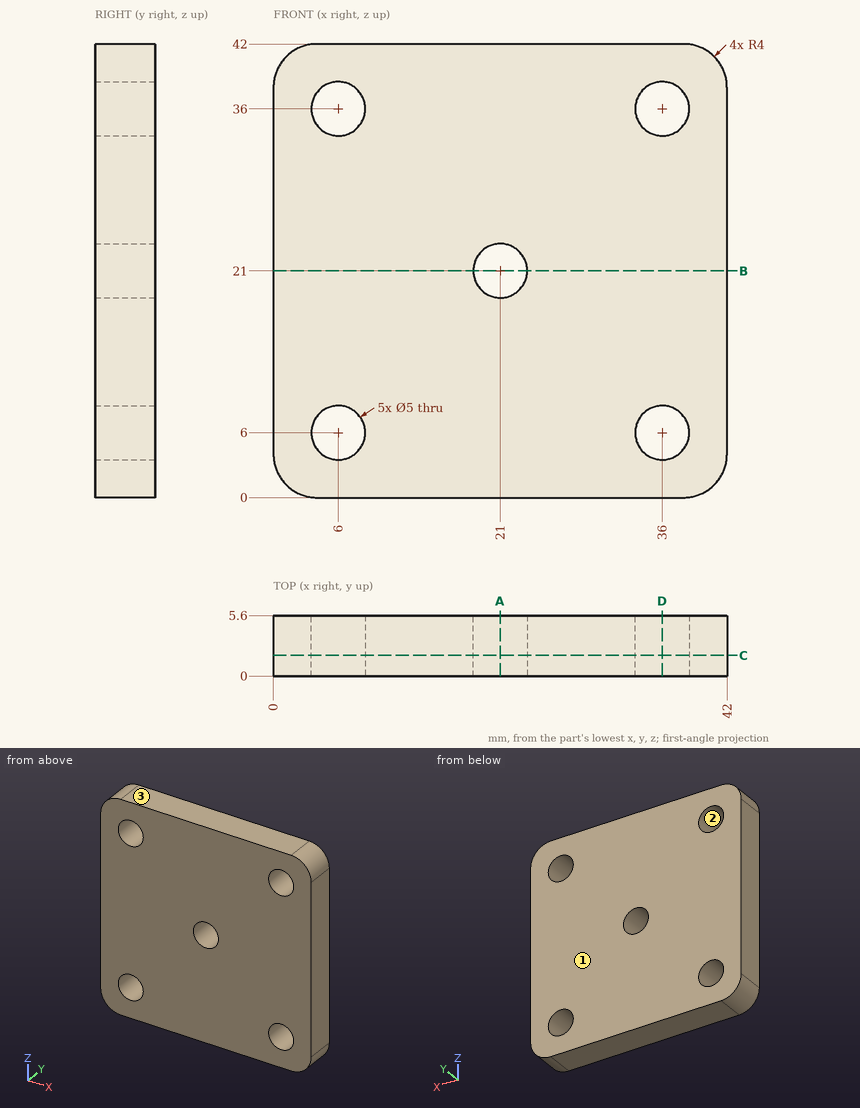
The figure shows three views and two pictorial views of one solid part (mm, origin at its lowest corner). Answer the questions. Round coordinates to 2 decimals unless told otherwise and drop trailing zeros. Write each loop counter-clockwise with the first axis right and the second up, starting at its lowest first coordinate (ties: lowest second). Pieces come first, ordered by that corner, then holes. Notation, with made-up numbers: M 54.5,-25.5 L 66.5,-25.5 A15 cw 66.5,-10.5 Z; hole C 75.25,-40 d10. An arc over 180 degrees is marked long. Use a Markdown table: item, result.
1) The part is cut by section D-D on x = 36. Give the vertices of the cut face in (y, z).
Taken from the geometry:
| item | result |
|---|---|
| outline | M 0,0 L 5.6,0 L 5.6,3.5 L 0,3.5 Z; M 0,8.5 L 5.6,8.5 L 5.6,33.5 L 0,33.5 Z; M 0,38.5 L 5.6,38.5 L 5.6,42 L 0,42 Z |
2) Determine the mould class of the marked faces 1, 2 and 3 for opening direction Z: pulls with the +Z half, pulls with the -Z half, needs draft (parallel to the pull), parting line crosses it, or undercut.
Taken from the geometry:
| item | result |
|---|---|
| face 1 | needs draft |
| face 2 | undercut |
| face 3 | pulls with the +Z half |
3) The part is cut by section C-C on y = 1.9. Give the vertices of the cut face in (x, z), plus the area to 3 significant figures.
Taken from the geometry:
| item | result |
|---|---|
| outline | M 0,4 A4 ccw 4,0 L 38,0 A4 ccw 42,4 L 42,38 A4 ccw 38,42 L 4,42 A4 ccw 0,38 Z; hole C 6,6 d5; hole C 6,36 d5; hole C 21,21 d5; hole C 36,6 d5; hole C 36,36 d5 |
| area | 1,650 mm2 |
4) Consider line 1 (Z direction, x = 36, y = 4.65); line 2 (X direction, y = 0.85, z = 8); line 3 (Z direction, x = 21, y = 4.45). Determine where each line is inside the solid, lowest interval first. Write a range as [from, to].
Taken from the geometry:
| item | result |
|---|---|
| line 1 | z = [0, 3.5], [8.5, 33.5], [38.5, 42] |
| line 2 | x = [0, 4.5], [7.5, 34.5], [37.5, 42] |
| line 3 | z = [0, 18.5], [23.5, 42] |
5) Flat-ended cylindrical pins translate along their axes: pin 1 (4 mm diameter, centred on x = 6, z = 6, fed in from -Y); pin 2 (6 mm diameter, centred on x = 37.5, z = 8, fed in from -Y). Find the tip coordinate at first contact, or state that the pin passes through.
Taken from the geometry:
| item | result |
|---|---|
| pin 1 | passes through |
| pin 2 | stops at y = 0 |
6) The part is cut by section B-B on z = 21. Give the vertices of the cut face in (x, y).
Taken from the geometry:
| item | result |
|---|---|
| outline | M 0,0 L 18.5,0 L 18.5,5.6 L 0,5.6 Z; M 23.5,0 L 42,0 L 42,5.6 L 23.5,5.6 Z |
7) The part is cut by section A-A on x = 21. Give the vertices of the cut face in (y, z).
Taken from the geometry:
| item | result |
|---|---|
| outline | M 0,0 L 5.6,0 L 5.6,18.5 L 0,18.5 Z; M 0,23.5 L 5.6,23.5 L 5.6,42 L 0,42 Z |
